Input: part model. Units: mm. Frame: model coordinates. Give positions to 0.01 mm unless a question says otherwise; leave off trailing zeros. Loops run counter-clockwise (first coordinate to the right, second up) from the corner with the lowest first, then second, coordinate; pieces in that order, holes last. Notation, with made-up numbers: (36, 19) -> (78, 19) arc R23 ccw to (78, 35) -> close; hole circle Ø8 at (24.5, 65.25). An arc over 180 degrees is marked (long way). Use CSV: the item, a comma, the result in double quotes.
```python
from build123d import *

# Parameters (mm, degrees)
SKETCH1_R                      = 21.275
BOSS_EXTRUDE1_DEPTH            = 3.175
M8_CLEARANCE_HOLE1_AT_2_COUNT  = 2
M8_CLEARANCE_HOLE1_AT_2_PITCH  = 81.35
SKETCH9_W                      = 125.35
SKETCH9_H                      = 8
SKETCH9_H_2                    = 2.5
BOSS_EXTRUDE2_DEPTH            = 3.175
M4_CLEARANCE_HOLE1_D           = 4.5
M4_CLEARANCE_HOLE1_CSINK_D     = 4.55
M4_CLEARANCE_HOLE1_CSINK_ANGLE = 90


with BuildPart() as part:
    # Sketch1 → Boss-Extrude1 (new body)
    with BuildSketch(Plane(origin=(0, 0, 0), x_dir=(1, 0, 0), z_dir=(0, 1, 0))):
        Polygon((-64, 0), (-64, 34), (61.35, 34), (61.35, 0), (61.35, -31.35), (-64, -31.35), align=None)
        with Locations(Location((0, 0, 0), (0, 0, 270))):
            Circle(SKETCH1_R, mode=Mode.SUBTRACT)
    extrude(amount=BOSS_EXTRUDE1_DEPTH)

    # Sketch4 → M8 Clearance Hole1 (revolve, cut)
    with BuildSketch(Plane(origin=(-42, 3.175, 0), x_dir=(0, 0, 1), z_dir=(1, 0, 0))):
        Polygon((0, 0), (0, 3.175), (4.5, 3.175), (4.5, 0.025), (4.525, 0), align=None)
    m8_clearance_hole1 = revolve(axis=Axis((-42, 9.525, 0), (0, -1, 0)), mode=Mode.SUBTRACT)

    # M8 Clearance Hole1 at 2: M8 Clearance Hole1 ×2
    with Locations(*[(i * M8_CLEARANCE_HOLE1_AT_2_PITCH, 0, 0) for i in range(1, M8_CLEARANCE_HOLE1_AT_2_COUNT)]):
        add(m8_clearance_hole1, mode=Mode.SUBTRACT)

    # Sketch9 → Boss-Extrude2 (add)
    with BuildSketch(Plane(origin=(0, 3.175, 0), x_dir=(1, 0, 0), z_dir=(0, 1, 0))):
        with Locations((-1.325, 38)):
            Rectangle(SKETCH9_W, SKETCH9_H)
        with Locations((-1.325, -32.6)):
            Rectangle(SKETCH9_W, SKETCH9_H_2)
    extrude(amount=-BOSS_EXTRUDE2_DEPTH)

    # M4 Clearance Hole1 (through all)
    with Locations(Plane(origin=(0, 3.175, 0), x_dir=(1, 0, 0), z_dir=(0, 1, 0))):
        with Locations((-56.35, 36.38795554), (-56.35, -26.35), (56.35, -26.35), (56.35, 36.38795554)):
            CounterSinkHole(M4_CLEARANCE_HOLE1_D / 2, M4_CLEARANCE_HOLE1_CSINK_D / 2, counter_sink_angle=M4_CLEARANCE_HOLE1_CSINK_ANGLE)


solid = part.part
```
1) Mould query, pull axis X, two halves, no side actions, for faces 1 (the flat face through (-2, 2, -42)), 2 (the flat face through (61.35, 2, -4)), 3 (the cylindrical face through (-58.496, 1.553, -37.064)). Classes: pulls with the +X half, pulls with the -X half, needs draft (parallel to the pull), parting line crosses it, or undercut.
From the geometry:
face 1,"needs draft"
face 2,"pulls with the +X half"
face 3,"undercut"
2) Ray query, line 1 (Z direction, x = -56.35, y = 1.9); line 2 (X direction, y = 2, z = 26.35); line 3 (X direction, y = 2.15, z = 0) (3 decimals). Return the intervals inside material, ascending.
From the geometry:
line 1,"z = -42 to -38.64, -34.14 to 24.1, 28.6 to 33.85"
line 2,"x = -64 to -58.6, -54.1 to 54.1, 58.6 to 61.35"
line 3,"x = -64 to -46.5, -37.5 to -21.275, 21.275 to 34.85, 43.85 to 61.35"
3) Section query C-C (x = 0). Return loops of the section in (y, z) (3 decimals), then the cut area to 3 significant figures.
From the geometry:
outline,"(0, -42) -> (3.175, -42) -> (3.175, -21.275) -> (0, -21.275) -> close; (0, 21.275) -> (3.175, 21.275) -> (3.175, 33.85) -> (0, 33.85) -> close"
area,"106 mm^2"
4) Contact query for flat-ended pins moving along their axis: pin 1 (1.5 mm diameter, centred on x = -24.5, z = 19, fed in from -Y); pin 2 (7 mm diameter, centred on x = -42, z = 0, fed in from -Y). Output: stop coordinate, or through.
From the geometry:
pin 1,"stops at y = 0"
pin 2,"passes through"
5) Section query D-D (z = -10.5). Return loops of the section in (x, y) (3 decimals), then the cut area to 3 significant figures.
From the geometry:
outline,"(-64, 0) -> (-18.503, 0) -> (-18.503, 3.175) -> (-64, 3.175) -> close; (18.503, 0) -> (61.35, 0) -> (61.35, 3.175) -> (18.503, 3.175) -> close"
area,"280 mm^2"
6) Section query A-A (z = 0). Return loops of the section in (x, y) (3 decimals).
From the geometry:
outline,"(-64, 0) -> (-46.5, 0) -> (-46.5, 3.15) -> (-46.525, 3.175) -> (-64, 3.175) -> close; (-37.5, 0) -> (-21.275, 0) -> (-21.275, 3.175) -> (-37.475, 3.175) -> (-37.5, 3.15) -> close; (21.275, 0) -> (34.85, 0) -> (34.85, 3.15) -> (34.825, 3.175) -> (21.275, 3.175) -> close; (43.85, 0) -> (61.35, 0) -> (61.35, 3.175) -> (43.875, 3.175) -> (43.85, 3.15) -> close"
7) Section query B-B (x = -56.35). Return loops of the section in (y, z) (3 decimals).
From the geometry:
outline,"(0, -42) -> (3.175, -42) -> (3.175, -38.663) -> (3.15, -38.638) -> (0, -38.638) -> close; (0, -34.138) -> (3.15, -34.138) -> (3.175, -34.113) -> (3.175, 24.075) -> (3.15, 24.1) -> (0, 24.1) -> close; (0, 28.6) -> (3.15, 28.6) -> (3.175, 28.625) -> (3.175, 33.85) -> (0, 33.85) -> close"
